Build history of the part. All positions in model axes, mm. A direction names the side the tool comes from. Give positions to 0.01 mm unless a question says otherwise; leave off trailing zeros. Loops run counter-clockwise (first coordinate to the right, second up) from the corner with the lowest first, then second, coordinate; pieces in that order, holes last. Notation, with made-up numbers: (20.25, 43.25) -> (44.25, 43.25) arc R33 ccw to (44.25, 74.25) -> close; hole circle Ø5 at (40.25, 11). An arc over 180 degrees is marked (long way). Answer as a JSON object with one key per item and string values. Group by question number.
from build123d import *

# Parameters (mm, degrees)
EXTRUDE_1_DEPTH    = 10
HOLE_WIZARD_M4_1_D = 3.3


with BuildPart() as part:
    # 草图1 → 凸台-拉伸1 (new body)
    with BuildSketch(Plane.XY):
        with BuildLine():
            Line((3, 3), (-3, 3))
            Line((-3, 3), (-3, 1.5))
            Line((-3, 1.5), (-4.666746731, 1.5))
            Line((-4.666746731, 1.5), (-4.666746731, 0.5))
            ThreePointArc((-4.666746731, 0.5), (-4.068683171, -1.006990331), (-2.6, -1.69377241))
            Line((-2.6, -1.69377241), (2.6, -1.69377241))
            ThreePointArc((2.6, -1.69377241), (4.068683171, -1.006990331), (4.666746731, 0.5))
            Line((4.666746731, 0.5), (4.666746731, 1.5))
            Line((4.666746731, 1.5), (3, 1.5))
            Line((3, 1.5), (3, 3))
        make_face()
    extrude(amount=EXTRUDE_1_DEPTH)

    # M4 螺纹孔1 (through all)
    with Locations(Plane(origin=(0, 3, 0), x_dir=(1, 0, 0), z_dir=(0, 1, 0))):
        with Locations((0, -5)):
            Hole(HOLE_WIZARD_M4_1_D / 2)


with BuildPart() as part_1:
    # Move Body 1: moved
    add(part.part.moved(Location((0, 0, -5))))


solid = part_1.part
(1) Saw through at A-A on x = 0. List the corners of the cut face in (y, z), plus the area to 3 significant figures.
(2) Saw through at C-C on y = 2.05. List the corners of the cut face in (x, z).
(3) Saw through at B-B on z = 0. List the corners of the cut face in (x, y), plus the area to 3 significant figures.
(4) Pin check, flat tips, straight feed: pin 1 (0.8 mm diameter, centred on y = 2, z = -0.5, fed in from -X); pin 2 (5.5 mm diameter, centred on x = 0, z = 0, fed in from +Y); pin 3 (0.8 mm diameter, centred on x = 4, z = 0.5, fed in from +Y); pin 4 (1.6 mm diameter, centred on y = 2.5, z = -0.5, fed in from +X). Stop position of each tip, or through.
(5) Probe line 1 along Z through (x, y) = (0, 0.65); line 2 along X through (y, z) = (0.9, 0); line 3 along X through (y, z) = (0, 0). List the from-to ranges inside material, lowest first. Write a range as [from, to].
(6) 3-axis set-ups, long thin cutter, end or side, ignore diameter. For faces 1 (the flat face through (4, 1.5, 0)), 2 (the flat face through (4.667, 1, 0)), 3 (the flat face through (-4, 1.5, 0)): which of +Z, -Z, +X, -X, +Y, -Y reach the whole face in a straight line?
(7) Saw through at D-D on z = -2.5. List the corners of the cut face in (x, y), plus the area to 3 significant figures.
(8) Pull direction Z, two halves, no side cores. Call faces 4 (the flat face through (0, 1, -5)), 5 (the cylindrical face through (1.216, 0.62, -1.115)), 6 (the flat face through (3, 2, 0)), 7 (the flat face through (0, 1, 5)): pulls with the +Z half, pulls with the -Z half, needs draft (parallel to the pull), parting line crosses it, or undercut.
Calculated:
{
 "1": {"outline": "(-1.69, -5) -> (3, -5) -> (3, -1.65) -> (-1.69, -1.65) -> close; (-1.69, 1.65) -> (3, 1.65) -> (3, 5) -> (-1.69, 5) -> close", "area": "31.4 mm^2"},
 "2": {"outline": "(-3, -5) -> (3, -5) -> (3, 5) -> (-3, 5) -> close; hole circle Ø3.3 at (0, 0)"},
 "3": {"outline": "(-4.67, 0.5) arc R2.2 ccw to (-2.6, -1.69) -> (-1.65, -1.69) -> (-1.65, 3) -> (-3, 3) -> (-3, 1.5) -> (-4.67, 1.5) -> close; (1.65, -1.69) -> (2.6, -1.69) arc R2.2 ccw to (4.67, 0.5) -> (4.67, 1.5) -> (3, 1.5) -> (3, 3) -> (1.65, 3) -> close", "area": "21.3 mm^2"},
 "4": {"pin 1": "stops at x = -3", "pin 2": "stops at y = 3", "pin 3": "stops at y = 1.5", "pin 4": "stops at x = 3"},
 "5": {"line 1": "z = [-5, -1.65], [1.65, 5]", "line 2": "x = [-4.67, -1.65], [1.65, 4.67]", "line 3": "x = [-4.61, -1.65], [1.65, 4.61]"},
 "6": {"face 1": "+Z, -Z, +X, +Y", "face 2": "+Z, -Z, +X, +Y, -Y", "face 3": "+Z, -Z, -X, +Y"},
 "7": {"outline": "(-4.67, 0.5) arc R2.2 ccw to (-2.6, -1.69) -> (2.6, -1.69) arc R2.2 ccw to (4.67, 0.5) -> (4.67, 1.5) -> (3, 1.5) -> (3, 3) -> (-3, 3) -> (-3, 1.5) -> (-4.67, 1.5) -> close", "area": "36.8 mm^2"},
 "8": {"face 4": "pulls with the -Z half", "face 5": "undercut", "face 6": "needs draft", "face 7": "pulls with the +Z half"}
}
